from build123d import *

# Parameters (mm, degrees)
SKETCH1_R                  = 4
BOSS_EXTRUDE1_DEPTH        = 51.562
SKETCH2_W                  = 0.444
SKETCH2_H                  = 0.762
CHAMFER2_SIZE              = 1
F_10_32_TAPPED_HOLE2_D     = 4.0386
F_10_32_TAPPED_HOLE2_DEPTH = 12.7
F_10_32_TAPPED_HOLE2_TIP   = 1.213317848


with BuildPart() as part:
    # Sketch1 → Boss-Extrude1 (new body)
    with BuildSketch(Plane.XY):
        Circle(SKETCH1_R)
    extrude(amount=BOSS_EXTRUDE1_DEPTH)

    # Sketch2 → Cut-Revolve1 (revolve, cut)
    with BuildSketch(Plane(origin=(0, 0, 0), x_dir=(1, 0, 0), z_dir=(0, 1, 0)), mode=Mode.PRIVATE) as cut_revolve1_sk:
        with Locations((3.778, -48.086)):
            Rectangle(SKETCH2_W, SKETCH2_H)
    revolve(cut_revolve1_sk.sketch.rotate(Axis((0, 0, 0), (0, 0, 1)), 180), axis=Axis((0, 0, 0), (0, 0, 1)), mode=Mode.SUBTRACT)

    # Chamfer2
    chamfer2_edges = [part.edges().sort_by_distance(p)[0] for p in [
        (-4, 0, 51.562),
    ]]
    chamfer(chamfer2_edges, length=CHAMFER2_SIZE)

    # #10-32 Tapped Hole2
    with Locations(Plane(origin=(0, 0, 0), x_dir=(-1, 0, 0), z_dir=(0, 0, -1))):
        with Locations((0, 0)):
            Hole(F_10_32_TAPPED_HOLE2_D / 2, depth=F_10_32_TAPPED_HOLE2_DEPTH)
            with Locations((0, 0, -(F_10_32_TAPPED_HOLE2_DEPTH + F_10_32_TAPPED_HOLE2_TIP / 2))):  # 118° drill point
                Cone(0, F_10_32_TAPPED_HOLE2_D / 2, F_10_32_TAPPED_HOLE2_TIP, mode=Mode.SUBTRACT)


solid = part.part
Input: part model. Units: mm. Frame: model coordinates. A direction names the side the tool comes from. Round coordinates to 2 decimals unless told otherwise and drop trailing zeros. Order: outer loops, then holes, each group sorted by start corner. A loop starts at its lowest first (then second) coordinate and runs counter-clockwise, first axis right, second up. Notation, with made-up numbers: (42.5, -1.5) - (50.5, -1.5) arc R10 cw to (50.5, 4.5) - close; hole circle Ø3 at (41.25, 17). An arc over 180 degrees is marked (long way). Answer as a JSON object with one key per item and string values. Group by question number.
(1) Cut plane A-A (z = 11). Return loops of the section in (x, y).
(2) Pin query (flat end, axial travel): P1, Ø3, axis at y = -2, z = 10, coming from the +X side. Return the tip coordinate at first contact, or that it passes through.
(3) Material intervals for probe 1 along Y at (x, z) = (0, 9); probe 2 along Z at (x, y) = (-2, 3.25) (3 decimals), sorted ascending. Write a range as from..to.
(4) Draft query along Y for faces 1 (the face through (-0.867, -3.905, 23.519)), 2 (the face through (0, 0, 51.562)), 3 (the face through (1.926, 0.607, 6.439)). Return one class per face: released by +Y, released by -Y, zero draft, split by the parting line, or undercut.
(5) Reachability of faces 4 (the face through (0.77, 3.47, 48.08)), 5 (the face through (-0.867, -3.905, 49.5)) from +Z, -Z, +X, -X, +Y, -Y: full face, straight path, thin tool, end or side. Return the list, or none.
(6) Cut plane B-B (z = 46). Return loops of the section in (x, y), then the cut area to 3 significant figures.
Here are the results:
{
 "1": {"outline": "circle Ø8 at (0, 0); hole circle Ø4.04 at (0, 0)"},
 "2": {"P1": "stops at x = 3.97"},
 "3": {"probe 1": "y = -4..-2.02, 2.02..4", "probe 2": "z = 0..47.705, 48.467..50.746"},
 "4": {"face 1": "split by the parting line", "face 2": "zero draft", "face 3": "undercut"},
 "5": {"face 4": "none", "face 5": "+Z, -Z"},
 "6": {"outline": "circle Ø8 at (0, 0)", "area": "50.3 mm^2"}
}
